Check sheet for the modelled part. Datum: model origin and axes. Units: mm. A direction names the side the tool comes from. Coordinates: 2 decimals unless noted, no trailing zeros. Order: outer loops, then holes, each group sorted by start corner. A loop starts at its lowest first (then second) coordinate and runs counter-clockwise, first axis right, second up.
from build123d import *

# Parameters (mm, degrees)
SKETCH5_R           = 6.35
BOSS_EXTRUDE2_DEPTH = 12.7
BOSS_EXTRUDE3_DEPTH = 31.75
CUT_EXTRUDE1_DEPTH  = 63.5
SKETCH10_R          = 3.175
CUT_EXTRUDE2_DEPTH  = 63.5


with BuildPart() as part:
    # Sketch5 → Boss-Extrude2 (new body)
    with BuildSketch(Plane(origin=(0, 0, 0), x_dir=(1, 0, 0), z_dir=(0, 1, 0))):
        with BuildLine():
            Line((-63.5, 25.4), (63.5, 25.4))
            ThreePointArc((63.5, 25.4), (88.9, 0), (63.5, -25.4))
            Line((63.5, -25.4), (-63.5, -25.4))
            ThreePointArc((-63.5, -25.4), (-88.9, 0), (-63.5, 25.4))
        make_face()
        with Locations((-63.5, 0)):
            Circle(SKETCH5_R, mode=Mode.SUBTRACT)
        with Locations((63.5, 0)):
            Circle(SKETCH5_R, mode=Mode.SUBTRACT)
    extrude(amount=BOSS_EXTRUDE2_DEPTH)

    # Sketch6 → Boss-Extrude3 (add, symmetric)
    with BuildSketch(Plane.XY):
        with BuildLine():
            Line((-41.275, 0), (41.275, 0))
            ThreePointArc((41.275, 0), (0, 41.275), (-41.275, 0))
        make_face()
    extrude(amount=BOSS_EXTRUDE3_DEPTH, both=True)

    # Sketch7 → Cut-Extrude1 (cut)
    with BuildSketch(Plane.XY.offset(31.75)):
        with BuildLine():
            Line((-31.75, 0), (31.75, 0))
            ThreePointArc((31.75, 0), (0, 31.75), (-31.75, 0))
        make_face()
    extrude(amount=-CUT_EXTRUDE1_DEPTH, mode=Mode.SUBTRACT)

    # Sketch10 → Cut-Extrude2 (cut)
    with BuildSketch(Plane(origin=(0, 41.275, 0), x_dir=(1, 0, 0), z_dir=(0, 1, 0))):
        Circle(SKETCH10_R)
    extrude(amount=-CUT_EXTRUDE2_DEPTH, mode=Mode.SUBTRACT)


solid = part.part
(1) Release check for a two-part mould opening along X. For faces 4 (the flat face through (51, 6, -25.4)), 5 (the cylindrical face through (88.894, 6.261, -0.559)), 6 (the cylindrical face through (-0.69, 36.5, 3.1)) record: +X half, -X half, draft (parallel to the pull), parting line (faces both ways), or undercut.
Filled in:
face 4: draft
face 5: +X half
face 6: undercut
(2) Thickness scan on probe 1 along Z at (x, y) = (0, 34) (3 decimals); probe 2 along Z at (x, y) = (-63, 4); probe 3 along X at (y, z) = (4, 0). Record the ranges inside material, lowest first.
Filled in:
probe 1: z = -31.75 to -3.175, 3.175 to 31.75
probe 2: z = -25.4 to -6.33, 6.33 to 25.4
probe 3: x = -88.9 to -69.85, -57.15 to -31.5, 31.5 to 57.15, 69.85 to 88.9
(3) Cross-section at C-C (z = 0). Enter the section's corners in (x, y) (3 decimals), and give its area (3 significant figures).
Filled in:
outline: (-88.9, 0) - (-69.85, 0) - (-69.85, 12.7) - (-88.9, 12.7) - close; (-57.15, 0) - (-31.75, 0) arc R31.75 cw to (-3.175, 31.591) - (-3.175, 41.153) arc R41.275 ccw to (-39.273, 12.7) - (-57.15, 12.7) - close; (3.175, 31.591) arc R31.75 cw to (31.75, 0) - (57.15, 0) - (57.15, 12.7) - (39.273, 12.7) arc R41.275 ccw to (3.175, 41.153) - close; (69.85, 0) - (88.9, 0) - (88.9, 12.7) - (69.85, 12.7) - close
area: 1,940 mm2
(4) Go/stop test with flat-tipped pins: P1, Ø12, axis at x = 46.5, z = 7.5, coming from the +Y side; P2, Ø14, axis at x = -56.5, y = 8.5, coming from the -Z side; P3, Ø8, axis at x = 15.5, y = 23.5, coming from the -Z side; P4, Ø7.5, axis at x = -63.5, z = 0, coming from the +Y side. Record where each tip stops, or that it passes through.
Filled in:
P1: stops at y = 12.7
P2: stops at z = -25.4
P3: stops at z = -31.75
P4: passes through
(5) Cross-section at D-D (z = -23.5). Enter the section's corners in (x, y) (3 decimals).
Filled in:
outline: (-73.139, 0) - (-31.75, 0) arc R31.75 cw to (31.75, 0) - (73.139, 0) - (73.139, 12.7) - (39.273, 12.7) arc R41.275 ccw to (-39.273, 12.7) - (-73.139, 12.7) - close
(6) Tool access check on faces 1 (the flat face through (-58, 12.7, 5)), 2 (the cylindrical face through (0.698, 31.742, 7.5)), 3 (the flat face through (59, 12.7, 5)). Record the directions out of +Z, -Z, +X, -X, +Y, -Y that give a thin tool (end or side, any length) a straight path to the whole face; none if there is none.
Filled in:
face 1: +Z, -Z, -X, +Y
face 2: +Z, -Z, -Y
face 3: +Z, -Z, +X, +Y
(7) Cross-section at A-A (y = 7). Enter the section's corners in (x, z).
Filled in:
outline: (-63.5, -25.4) - (-40.68, -25.4) - (-40.68, -31.75) - (-30.97, -31.75) - (-30.97, 31.75) - (-40.68, 31.75) - (-40.68, 25.4) - (-63.5, 25.4) arc R25.4 ccw to start; (30.97, -31.75) - (40.68, -31.75) - (40.68, -25.4) - (63.5, -25.4) arc R25.4 ccw to (63.5, 25.4) - (40.68, 25.4) - (40.68, 31.75) - (30.97, 31.75) - close; hole circle Ø12.7 at (-63.5, 0); hole circle Ø12.7 at (63.5, 0)
(8) Cross-section at B-B (x = 0). Enter the section's corners in (y, z) (3 decimals), and give its area (3 significant figures).
Filled in:
outline: (31.75, -31.75) - (41.275, -31.75) - (41.275, -3.175) - (31.75, -3.175) - close; (31.75, 3.175) - (41.275, 3.175) - (41.275, 31.75) - (31.75, 31.75) - close
area: 544 mm2
